Autodesk Inventor part; units mm, degrees
ref_plane "YZ Plane" through (0, 0, 0) normal (1, 0, 0) x (0, 1, 0)
ref_plane "XZ Plane" through (0, 0, 0) normal (0, 1, 0) x (-1, 0, 0)
ref_plane "XY Plane" through (0, 0, 0) normal (0, 0, 1) x (1, 0, 0)
sketch "Sketch1" plane through (0, 0, 0) normal (1, 0, 0) x (0, 1, 0)
  line L0 (0, -13.6) -> (0, 23.4)
  line L1 (0, 23.4) -> (2.5, 23.4)
  line L2 (2.5, 23.4) -> (2.5, 2)
  line L3 (2.5, 2) -> (4, 2)
  line L4 (4, 2) -> (4, 0)
  line L5 (4, 0) -> (2.5, 0)
  line L6 (2.5, 0) -> (2.5, -13.6)
  line L7 (2.5, -13.6) -> (0, -13.6)
  point P0 (0, 0)
  dimension "d0" = 5
  dimension "d1" = 37
  dimension "d2" = 13.6
  dimension "d3" = 2
  dimension "d4" = 8
revolve "Revolution1" add sketch "Sketch1" angle 360 about axis through (0, 0, -13.6) along (0, 0, 1)
chamfer "Chamfer1" distance 0.4 angle 45 2 edges at (0, -2.5, -13.6) (0, -2.5, 23.4)
chamfer "Chamfer2" distance 0.2 angle 45 2 edges at (0, -4, 2) (0, -4, 0)
properties part number "rail-shaft" material "Stainless Steel"
For this review, take the finished solid that the model builds, in its own axes (mm). A direction names the side the tool comes from. Round coordinates to 2 decimals unless told otherwise and drop trailing zeros. Loops run counter-clockwise (first coordinate to the right, second up) from the corner with the lowest first, then second, coordinate; pieces in that order, holes last. Notation, with made-up numbers: (68, 17) - (111, 17) arc R24 cw to (111, 28) - close; hole circle Ø11 at (0.5, 72.5). An arc over 180 degrees is marked (long way). Answer as CSV lines item,"result".
(1) Consider section C-C on z = 18. Give the boundary of the cut face in (x, y), then the cut area to 3 significant figures.
Checked values:
outline,"circle Ø5 at (0, 0)"
area,"19.6 mm2"
(2) Tool access review of faces 1 (the face through (2.5, -0.9, 2)), 2 (the face through (0, 0, -13.6)), 3 (the face through (2.5, -0.9, 0)): name each direction out of +Z, -Z, +X, -X, +Y, -Y from which nothing blocks a thin tool from reaching the whole face with its end or side.
Checked values:
face 1,"+Z"
face 2,"-Z, +X, -X, +Y, -Y"
face 3,"-Z"
(3) Consider section A-A on x = 0. Give the boundary of the cut face in (y, z), then the cut area to 3 significant figures.
Checked values:
outline,"(-4, 0.2) - (-3.8, 0) - (-2.5, 0) - (-2.5, -13.2) - (-2.1, -13.6) - (2.1, -13.6) - (2.5, -13.2) - (2.5, 0) - (3.8, 0) - (4, 0.2) - (4, 1.8) - (3.8, 2) - (2.5, 2) - (2.5, 23) - (2.1, 23.4) - (-2.1, 23.4) - (-2.5, 23) - (-2.5, 2) - (-3.8, 2) - (-4, 1.8) - close"
area,"191 mm2"
(4) Insertion check: P1, Ø1, axis at x = -2.5, z = 2, coming from the -Y side; P2, Ø4, axis at x = -2, z = -7.5, coming from the +Y side; P3, Ø1.5, axis at y = 1, z = 8, coming from the +X side. Each pin has a flat end and moves straight along its axis. Give the tip position at first contact, or say it passes through.
Checked values:
P1,"stops at y = -3.44"
P2,"stops at y = 2.5"
P3,"stops at x = 2.49"
(5) Wall thickness on line 1 (Z direction, x = 2, y = 2.5); line 2 (X direction, y = -1.5, z = 17.5); line 3 (X direction, y = 0.25, z = 17): over which ranges is each line inside the solid? List them lowest first.
Checked values:
line 1,"z = 0 to 2"
line 2,"x = -2 to 2"
line 3,"x = -2.49 to 2.49"
(6) Mouldability with a two-part tool opening along Y and no side actions: class faces 4 (the face through (0, 0, 23.4)), 5 (the face through (-2.44, -0.54, -6.69)) as +Y half, -Y half, draft (parallel to the pull), parting line (faces both ways), or undercut.
Checked values:
face 4,"draft"
face 5,"parting line"
